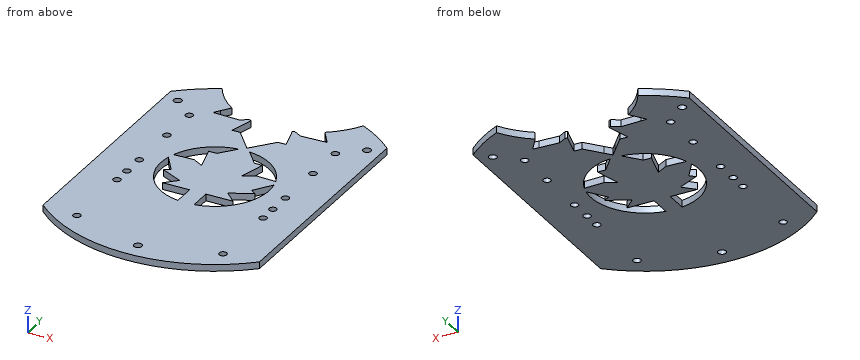
from build123d import *

# Parameters (mm, degrees)
SKETCH1_R           = 1.89865
BOSS_EXTRUDE3_DEPTH = 3.175
CUT_EXTRUDE2_DEPTH  = 3.175
SKETCH4_R           = 1.778
CUT_EXTRUDE3_DEPTH  = 3.175
SKETCH5_R           = 1.778
CUT_EXTRUDE4_DEPTH  = 3.175
CUT_EXTRUDE5_DEPTH  = 3.175


with BuildPart() as part:
    # Sketch1 → Boss-Extrude3 (new body)
    with BuildSketch(Plane.XY):
        with BuildLine():
            Line((-50.8, 55.175719298), (-50.8, -55.175719298))
            ThreePointArc((-50.8, -55.175719298), (0, -75), (50.8, -55.175719298))
            Line((50.8, -55.175719298), (50.8, 55.175719298))
            ThreePointArc((50.8, 55.175719298), (42.419210034, 61.851520758), (33.172661219, 67.264957799))
            ThreePointArc((33.172661219, 67.264957799), (0, 47.904876359), (-33.172661219, 67.264957799))
            ThreePointArc((-33.172661219, 67.264957799), (-42.419210034, 61.851520758), (-50.8, 55.175719298))
        make_face()
        with Locations((0, -66.675)):
            Circle(SKETCH1_R, mode=Mode.SUBTRACT)
        with Locations((-44.45, 49.6966108)):
            Circle(SKETCH1_R, mode=Mode.SUBTRACT)
        with Locations(Location((44.45, 49.6966108, 0), (0, 0, 180))):
            Circle(SKETCH1_R, mode=Mode.SUBTRACT)
    extrude(amount=BOSS_EXTRUDE3_DEPTH)

    # Sketch3 → Cut-Extrude2 (cut)
    with BuildSketch(Plane.XY.offset(3.175)):
        with BuildLine():
            Line((8.827105782, 17.78), (2.54, 25.272680903))
            ThreePointArc((2.54, 25.272680903), (15.758317518, 19.920728626), (24.009298775, 8.289365013))
            Line((24.009298775, 8.289365013), (14.484298775, 8.647939367))
            Line((14.484298775, 8.647939367), (9.404298775, 5.715))
            Line((9.404298775, 5.715), (12.637105782, 17.78))
            Line((12.637105782, 17.78), (8.827105782, 17.78))
        make_face()
        with BuildLine():
            Line((18.868143133, -3.140634987), (24.826209076, 5.368365013))
            ThreePointArc((24.826209076, 5.368365013), (20.911260009, -14.418016674), (3.81, -25.112624315))
            Line((3.81, -25.112624315), (3.81, -14.877877919))
            Line((3.81, -14.877877919), (16.51, -14.877877919))
            Line((16.51, -14.877877919), (11.327081569, -9.797877919))
            Line((11.327081569, -9.797877919), (21.487081569, -4.935568543))
            Line((21.487081569, -4.935568543), (18.868143133, -3.140634987))
        make_face()
        with BuildLine():
            Line((-3.81, -14.877877919), (-3.81, -25.112624315))
            ThreePointArc((-3.81, -25.112624315), (-20.911260009, -14.418016674), (-24.826209076, 5.368365013))
            Line((-24.826209076, 5.368365013), (-18.868143133, -3.140634987))
            Line((-18.868143133, -3.140634987), (-21.487081569, -4.935568543))
            Line((-21.487081569, -4.935568543), (-11.327081569, -9.797877919))
            Line((-11.327081569, -9.797877919), (-16.51, -14.877877919))
            Line((-16.51, -14.877877919), (-3.81, -14.877877919))
        make_face()
        with BuildLine():
            Line((-14.484298775, 8.647939367), (-24.009298775, 8.289365013))
            ThreePointArc((-24.009298775, 8.289365013), (-15.758317518, 19.920728626), (-2.54, 25.272680903))
            Line((-2.54, 25.272680903), (-8.827105782, 17.78))
            Line((-8.827105782, 17.78), (-12.637105782, 17.78))
            Line((-12.637105782, 17.78), (-9.404298775, 5.715))
            Line((-9.404298775, 5.715), (-14.484298775, 8.647939367))
        make_face()
    extrude(amount=-CUT_EXTRUDE2_DEPTH, mode=Mode.SUBTRACT)

    # Sketch4 → Cut-Extrude3 (cut)
    with BuildSketch(Plane.XY.offset(3.175)):
        with Locations((-34.29, 40.919876359)):
            Circle(SKETCH4_R)
        with Locations((34.29, 40.919876359)):
            Circle(SKETCH4_R)
        with Locations((34.29, -2.260123641)):
            Circle(SKETCH4_R)
        with Locations((-34.29, -2.260123641)):
            Circle(SKETCH4_R)
        with Locations((-34.29, -13.055123641)):
            Circle(SKETCH4_R)
        with Locations((34.29, -13.055123641)):
            Circle(SKETCH4_R)
        with Locations((34.29, -56.235123641)):
            Circle(SKETCH4_R)
        with Locations((-34.29, -56.235123641)):
            Circle(SKETCH4_R)
    extrude(amount=-CUT_EXTRUDE3_DEPTH, mode=Mode.SUBTRACT)

    # Sketch5 → Cut-Extrude4 (cut)
    with BuildSketch(Plane.XY.offset(3.175)):
        with Locations((-34.29, 21.59)):
            Circle(SKETCH5_R)
        with Locations((34.29, 21.59)):
            Circle(SKETCH5_R)
        with Locations((34.29, -21.59)):
            Circle(SKETCH5_R)
        with Locations((-34.29, -21.59)):
            Circle(SKETCH5_R)
    extrude(amount=-CUT_EXTRUDE4_DEPTH, mode=Mode.SUBTRACT)

    # Sketch6 → Cut-Extrude5 (cut)
    with BuildSketch(Plane.XY.offset(3.175)):
        Polygon((-8.827105782, 38.1), (-2.54, 30.607319097), (0, 27.580264972), (2.54, 30.607319097), (8.827105782, 38.1), (12.637105782, 38.1), (9.404298775, 50.165), (14.484298775, 47.232060633), (24.009298775, 47.590634987), (26.798005722, 47.695617537), (24.826209076, 50.511634987), (18.868143133, 59.020634987), (-18.868143133, 59.020634987), (-24.826209076, 50.511634987), (-26.798005722, 47.695617537), (-24.009298775, 47.590634987), (-14.484298775, 47.232060633), (-9.404298775, 50.165), (-12.637105782, 38.1), align=None)
    extrude(amount=-CUT_EXTRUDE5_DEPTH, mode=Mode.SUBTRACT)


solid = part.part
Geometry check sheet. Reference: the model listing, model coordinates, mm. Round coordinates to 2 decimals unless told otherwise and drop trailing zeros. Loops run counter-clockwise (first coordinate to the right, second up) from the corner with the lowest first, then second, coordinate; pieces in that order, holes last. Notation, with made-up numbers: (45, 21) -> (95, 21) arc R18 ccw to (95, 40) -> close; hole circle Ø5 at (22, 47). An arc over 180 degrees is marked (long way). Answer as a JSON object with one key per item and string values. Group by question number.
Item 1: Thickness scan on line 1 along X through (y, z) = (45.5, 1.6); line 2 along X through (y, z) = (39.5, 2.95); line 3 along X through (y, z) = (15.5, 1.25). Record the ranges inside material, lowest first.
Item 2: Cross-section at B-B, the plane x = -44.45. Record the cut outline in (y, z) (3 decimals).
Item 3: Cross-section at A-A, the plane y = 21.59. Record the cut outline in (x, z) (3 decimals).
Item 4: Depth check by flat-ended pin: pin 1 Ø4 at (x, y) = (-34.29, -21.59) entering from -Z; pin 2 Ø1.6 at (x, z) = (11.5, 2.5) entering from +Y. Enter the tip coordinate at first touch or a pass-through.
Item 5: Cross-section at C-C, the plane z = 1.65. Count the separate pieces of the cut face and the enclosed holes in it, plus the area to 3 significant figures.
Determined:
{
 "1": {"line 1": "x = -50.8 to -10.65, 10.65 to 50.8", "line 2": "x = -50.8 to -35.36, -33.22 to -12.26, 12.26 to 33.22, 35.36 to 50.8", "line 3": "x = -50.8 to -20.12, -12.03 to 12.03, 20.12 to 50.8"},
 "2": {"outline": "(-60.409, 0) -> (47.798, 0) -> (47.798, 3.175) -> (-60.409, 3.175) -> close; (51.595, 0) -> (60.409, 0) -> (60.409, 3.175) -> (51.595, 3.175) -> close"},
 "3": {"outline": "(-50.8, 0) -> (-36.068, 0) -> (-36.068, 3.175) -> (-50.8, 3.175) -> close; (-32.512, 0) -> (-13.38, 0) -> (-13.38, 3.175) -> (-32.512, 3.175) -> close; (-5.63, 0) -> (5.63, 0) -> (5.63, 3.175) -> (-5.63, 3.175) -> close; (13.38, 0) -> (32.512, 0) -> (32.512, 3.175) -> (13.38, 3.175) -> close; (36.068, 0) -> (50.8, 0) -> (50.8, 3.175) -> (36.068, 3.175) -> close"},
 "4": {"pin 1": "stops at z = 0", "pin 2": "stops at y = 49.42"},
 "5": {"separate pieces": "1", "enclosed holes": "19", "area": "11,400 mm²"}
}
